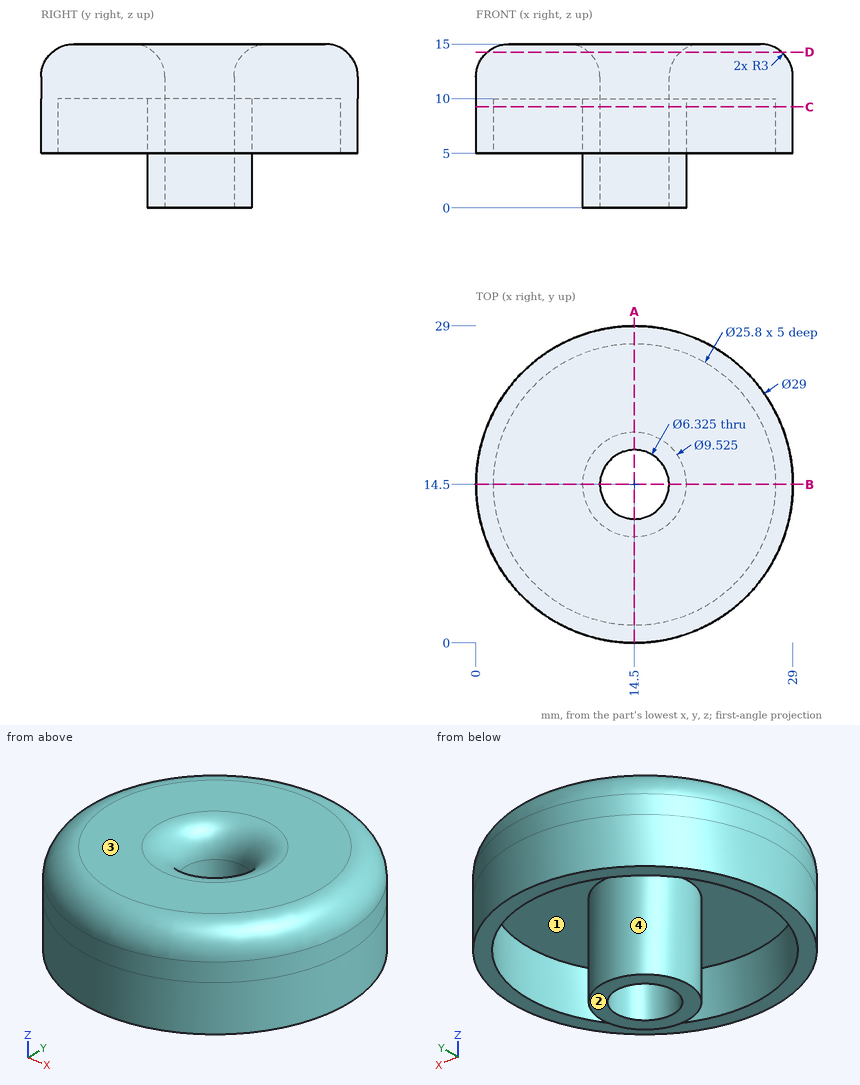
Source: three-view drawing plus pictorial views. Frame: mm from the lowest corner of the part. A direction names the side the tool comes from. Give positions to 0.01 mm unless a question says otherwise; leave off trailing zeros. Write each loop counter-clockwise with the first axis right and the second up, starting at its lowest first coordinate (ties: lowest second). Pieces come first, ordered by that corner, then holes. Notation, with made-up numbers: (-25, 60.25) -> (19, 60.25) arc R33 cw to (19, 99.25) -> close; hole circle Ø9 at (-1, -9.5). An arc over 180 degrees is marked (long way). Answer in a Markdown table with one row per item.
(1) Section query C-C on z = 9.25. Return loops of the section in (x, y) (1 decimal), then the cut area to 3 significant figures.
Answers below:
| item | result |
|---|---|
| outline | circle Ø29 at (14.5, 14.5); circle Ø9.5 at (14.5, 14.5); hole circle Ø25.8 at (14.5, 14.5); hole circle Ø6.3 at (14.5, 14.5) |
| area | 178 mm^2 |
(2) Section query A-A on x = 14.5. Return loops of the section in (y, z), then the cut area to 3 significant figures.
Answers below:
| item | result |
|---|---|
| outline | (0, 5) -> (1.6, 5) -> (1.6, 10) -> (9.74, 10) -> (9.74, 0) -> (11.34, 0) -> (11.34, 12) arc R3 ccw to (8.34, 15) -> (3, 15) arc R3 ccw to (0, 12) -> close; (17.66, 0) -> (19.26, 0) -> (19.26, 10) -> (27.4, 10) -> (27.4, 5) -> (29, 5) -> (29, 12) arc R3 ccw to (26, 15) -> (20.66, 15) arc R3 ccw to (17.66, 12) -> close |
| area | 154 mm^2 |
(3) Draft query along Y for the marked faces 1 and 2. Return one class per face: +Y half, -Y half, draft (parallel to the pull), parting line (faces both ways), or undercut.
Answers below:
| item | result |
|---|---|
| face 1 | undercut |
| face 2 | draft |
(4) Ray query, line 1 along Y through (x, z) = (14.5, 7.8); line 2 along Y through (x, z) = (15.75, 8); line 3 along X through (y, z) = (16.5, 5.5). Return the intervals inside material, ascending. Write a range as [from, to].
Answers below:
| item | result |
|---|---|
| line 1 | [0, 1.6], [9.74, 11.34], [17.66, 19.26], [27.4, 29] |
| line 2 | [0.05, 1.66], [9.9, 11.6], [17.4, 19.1], [27.34, 28.95] |
| line 3 | [0.14, 1.76], [10.18, 12.05], [16.95, 18.82], [27.24, 28.86] |
(5) Section query D-D on z = 14.25. Return loops of the section in (x, y).
Answers below:
| item | result |
|---|---|
| outline | circle Ø26.97 at (14.5, 14.5); hole circle Ø8.36 at (14.5, 14.5) |
(6) Pin query (flat end, axial travel): pin 1 (8 mm diameter, centred on y = 21, z = 11.5, fed in from +X); pin 2 (2 mm diameter, centred on x = 11.5, y = 23, fed in from -Z); pin 3 (4 mm diameter, centred on x = 17, y = 3.5, fed in from -Z). Return the tip coordinate at first contact, or that it passes through.
Answers below:
| item | result |
|---|---|
| pin 1 | x = 28.78 |
| pin 2 | z = 10 |
| pin 3 | z = 5 |
(7) Set-up query: the marked faces 3 and 4. Return all of +Z, -Z, +X, -X, +Y, -Y with unobstructed straight access to the full face (end or side cutting, diameter ignored); none if empty.
Answers below:
| item | result |
|---|---|
| face 3 | +Z, +X, -X, +Y, -Y |
| face 4 | -Z |
